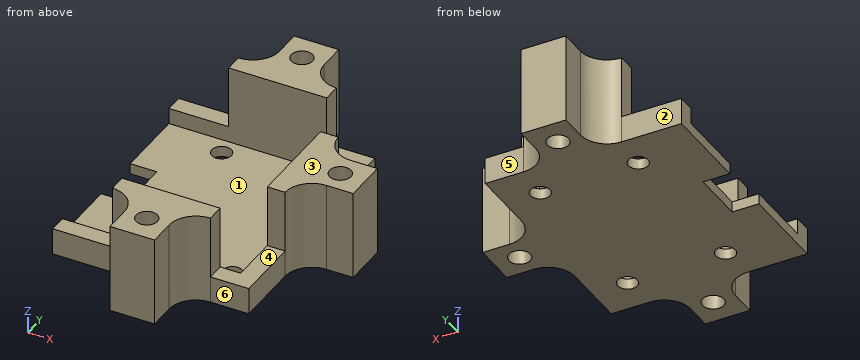
from build123d import *

# Parameters (mm, degrees)
SKETCH1_R           = 1.1
SKETCH1_W           = 5
SKETCH1_H           = 6
SKETCH1_R_2         = 1.2
SKETCH1_W_2         = 6
SKETCH1_H_2         = 5
BOSS_EXTRUDE1_DEPTH = 10
FILLET1_R           = 3
SKETCH2_W           = 28
SKETCH2_H           = 22
CUT_EXTRUDE1_DEPTH  = 8.8
SKETCH3_W           = 6.7
SKETCH3_H           = 26
SKETCH3_W_2         = 4.3
SKETCH3_H_2         = 7.5
CUT_EXTRUDE2_DEPTH  = 7


with BuildPart() as part:
    # Sketch1 → Boss-Extrude1 (new body)
    # profile 1 of 4: a face of its own
    with BuildSketch(Plane.XY):
        Polygon((0, 0), (22, 0), (22, -26), (0, -26), (0, -16), (3, -16), (3, -10), (0, -10), align=None)
        with Locations((18, -4)):
            Circle(SKETCH1_R, mode=Mode.SUBTRACT)
        with Locations((7, -4)):
            Circle(SKETCH1_R, mode=Mode.SUBTRACT)
        with Locations((7, -22)):
            Circle(SKETCH1_R, mode=Mode.SUBTRACT)
        with Locations((18, -22)):
            Circle(SKETCH1_R, mode=Mode.SUBTRACT)
    # profile 2 of 4: a face of its own
    with BuildSketch(Plane.XY):
        with Locations((12.2, 3)):
            Rectangle(SKETCH1_W, SKETCH1_H)
        with Locations((12.2, 3)):
            Circle(SKETCH1_R_2, mode=Mode.SUBTRACT)
    # profile 3 of 4: a face of its own
    with BuildSketch(Plane.XY):
        with Locations((25, -13)):
            Rectangle(SKETCH1_W_2, SKETCH1_H_2)
        with Locations((25.2, -13)):
            Circle(SKETCH1_R_2, mode=Mode.SUBTRACT)
    # profile 4 of 4: a face of its own
    with BuildSketch(Plane.XY):
        with Locations((12.2, -29)):
            Rectangle(SKETCH1_W, SKETCH1_H)
        with Locations((12.2, -29)):
            Circle(SKETCH1_R_2, mode=Mode.SUBTRACT)
    extrude(amount=BOSS_EXTRUDE1_DEPTH)

    # Fillet1
    fillet1_edges = [part.edges().sort_by_distance(p)[0] for p in [
        (9.7, 0, 5),
        (14.7, 0, 5),
        (22, -10.5, 5),
        (22, -15.5, 5),
        (14.7, -26, 5),
        (9.7, -26, 5),
    ]]
    fillet(fillet1_edges, radius=FILLET1_R)

    # Sketch2 → Cut-Extrude1 (cut)
    with BuildSketch(Plane.XY.offset(10)):
        with Locations((6, -13)):
            Rectangle(SKETCH2_W, SKETCH2_H)
    extrude(amount=-CUT_EXTRUDE1_DEPTH, mode=Mode.SUBTRACT)

    # Sketch3 → Cut-Extrude2 (cut)
    with BuildSketch(Plane.XY.offset(10)):
        with Locations((3.35, -13)):
            Rectangle(SKETCH3_W, SKETCH3_H)
        with Locations((19.85, -3.75)):
            Rectangle(SKETCH3_W_2, SKETCH3_H_2)
        with Locations((19.85, -22.25)):
            Rectangle(SKETCH3_W_2, SKETCH3_H_2)
    extrude(amount=-CUT_EXTRUDE2_DEPTH, mode=Mode.SUBTRACT)


solid = part.part
Can you work these out from the model? Positions are in its coordinate system, mm. Face numbers are marked on the shaded views. A direction names the side the tool comes from. Give positions to 0.01 mm unless a question says otherwise; leave off trailing zeros. Order: outer loops, then holes, each group sorted by start corner. A loop starts at its lowest first (then second) coordinate and runs counter-clockwise, first axis right, second up. Notation, with made-up numbers: M 57.25,-4.75 L 66.25,-4.75 A25 cw 66.25,9.25 Z; hole C 87.5,18 d9. An arc over 180 degrees is marked long. Use one line per item in the form item = value.
Item 1: If we section it at A-A, the plane z = 8: Write out the boundary of the cut face in (x, y), and give its area (3 significant figures).
Values follow:
outline = M 6.7,-26 A3 cw 9.7,-29 L 9.7,-32 L 14.7,-32 L 14.7,-29 A3 cw 17.7,-26 L 17.7,-24 L 6.7,-24 Z; M 6.7,-2 L 17.7,-2 L 17.7,0 A3 cw 14.7,3 L 14.7,6 L 9.7,6 L 9.7,3 A3 cw 6.7,0 Z; M 20,-18.5 L 22,-18.5 A3 cw 25,-15.5 L 28,-15.5 L 28,-10.5 L 25,-10.5 A3 cw 22,-7.5 L 20,-7.5 Z; hole C 12.2,-29 d2.4; hole C 12.2,3 d2.4; hole C 25.2,-13 d2.4
area = 154 mm^2
Item 2: For the marked faces 4, 5 and 6, which set-ups out of +Z, -Z, +X, -X, +Y, -Y let a thin tool reach every point of the face, with its end or its side?
Values follow:
face_4 = +Z, +X, -Y
face_5 = +Z, -Z, +X, +Y
face_6 = +Z, -Z, +X, -Y
Item 3: If we section it at B-B, the plane x = 12.2: Write out the boundary of the cut face in (y, z), and give its area (3 significant figures).
Values follow:
outline = M -32,0 L -30.2,0 L -30.2,10 L -32,10 Z; M -27.8,0 L 1.8,0 L 1.8,10 L -2,10 L -2,1.2 L -24,1.2 L -24,10 L -27.8,10 Z; M 4.2,0 L 6,0 L 6,10 L 4.2,10 Z
area = 138 mm^2
Item 4: Thinking about a two-plate mould opening in Y: for the marked faces 1, 2 and 3, which applies, pulls with the +Y half, pulls with the -Y half, needs draft (parallel to the pull), parting line crosses it, or undercut?
Values follow:
face_1 = undercut
face_2 = pulls with the +Y half
face_3 = needs draft
Item 5: If we section it at D-D, the plane y = 2.5: Write out the boundary of the cut face in (x, z).
Values follow:
outline = M 9.66,0 L 11.11,0 L 11.11,10 L 9.66,10 Z; M 13.29,0 L 14.74,0 L 14.74,10 L 13.29,10 Z
Item 6: Will these pins go through, and if not, where does the flat tip stop? pin 1 Ø3.5 at (x, y) = (20.5, -4) entering from +Z; pin 2 Ø1.6 at (x, z) = (21.5, 5) entering from -Y; pin 3 Ø1.6 at (y, z) = (-1, 7.5) entering from -X.
Values follow:
pin_1 = 3
pin_2 = -18.5
pin_3 = 6.7
Item 7: If I drill on line 1 along Y through (x, z) = (12.2, 3.75); line 2 along X through (y, z) = (-4, 0.4); line 3 along Y through (x, z) = (18, 0.85), over which ranges is the centre line in solid material (lowest first)? Write a range as [from, to].
Values follow:
line_1 = [-32, -30.2], [-27.8, -24], [-2, 1.8], [4.2, 6]
line_2 = [0, 5.9], [8.1, 16.9], [19.1, 22]
line_3 = [-26, -23.1], [-20.9, -5.1], [-2.9, 0]
Item 8: If we section it at C-C, the plane y = -4: Write out the boundary of the cut face in (x, z).
Values follow:
outline = M 0,0 L 5.9,0 L 5.9,1.2 L 0,1.2 Z; M 8.1,0 L 16.9,0 L 16.9,1.2 L 8.1,1.2 Z; M 19.1,0 L 22,0 L 22,3 L 20,3 L 20,1.2 L 19.1,1.2 Z
